Work out the finished part from the listing and answer in its coordinate system (mm). Face numbers are marked on the shaded views. A direction names the side the tool comes from. Coordinates: 2 decimals unless noted, no trailing zeros. Write each loop counter-clockwise with the first axis right and the second up, starting at its lowest first coordinate (ties: lowest second). Pieces come first, ordered by that corner, then holes. Notation, with made-up numbers: (-25, -35) - (12, -35) arc R17 cw to (12, -14) - close; hole circle Ø2 at (76.25, 65). An arc over 180 degrees is marked (long way). Use one line per item in the form item = value. Start each with the question number.
Item 1: A cutting plane is placed at B-B (y = 8). Write down the section's boundary in (x, z), then the cut area to 3 significant figures.
Item 2: Given pin 1 (5 mm diameter, centred on y = 4, z = 0.5, fed in from +X); pin 2 (5 mm diameter, centred on x = -0.5, y = 9, fed in from -Z); pin 3 (2 mm diameter, centred on y = 12.5, z = -3, fed in from +X), each flat-ended and moving along its own axis, determine where each tip first touches the part or whether it passes through.
Item 3: Consider probe 1 along Y at (x, z) = (-1.5, -3); probe 2 along Y at (x, z) = (0, 0.75); probe 3 along X at (y, z) = (6, -1.5). Determine where each line is inside the solid, lowest interval first.
Item 4: Determine the mould class of the marked faces 4, 5, 6 and 7 for opening direction X: released by +X, released by -X, zero draft, split by the parting line, or undercut.
Item 5: For the marked faces 1, 2 and 3, determine the directions among +Z, -Z, +X, -X, +Y, -Y from which every point of the face is accessible in a straight line to the end or side of a thin tool.
Item 6: A cutting plane is placed at A-A (z = 0). Write down the section's boundary in (x, y).
from build123d import *

# Parameters (mm, degrees)
SKETCH2_R           = 2.5
BOSS_EXTRUDE1_DEPTH = 30
SKETCH3_R           = 4.25
BOSS_EXTRUDE2_DEPTH = 5
FILLET1_R           = 0.4
CHAMFER1_SIZE       = 0.5
CUT_EXTRUDE1_DEPTH  = 2.5


with BuildPart() as part:
    # Sketch2 → Boss-Extrude1 (new body)
    with BuildSketch(Plane(origin=(0, 0, 0), x_dir=(1, 0, 0), z_dir=(0, 1, 0))):
        with Locations(Location((0, 0, 0), (0, 0, 270))):
            Circle(SKETCH2_R)
    extrude(amount=BOSS_EXTRUDE1_DEPTH)

    # Sketch3 → Boss-Extrude2 (add)
    with BuildSketch(Plane(origin=(0, 0, 0), x_dir=(1, 0, 0), z_dir=(0, 1, 0))):
        with Locations(Location((0, 0, 0), (0, 0, 270))):
            Circle(SKETCH3_R)
    extrude(amount=-BOSS_EXTRUDE2_DEPTH)

    # Fillet1
    fillet1_edges = [part.edges().sort_by_distance(p)[0] for p in [
        (0, 0, -2.5),
    ]]
    fillet(fillet1_edges, radius=FILLET1_R)

    # Chamfer1
    chamfer1_edges = [part.edges().sort_by_distance(p)[0] for p in [
        (0, 30, -2.5),
        (0, -5, -4.25),
    ]]
    chamfer(chamfer1_edges, length=CHAMFER1_SIZE)

    # Sketch4 → Cut-Extrude1 (cut)
    with BuildSketch(Plane.XZ.offset(5)):
        Polygon((0, 2.309401077), (-2, 1.154700538), (-2, -1.154700538), (0, -2.309401077), (2, -1.154700538), (2, 1.154700538), align=None)
    extrude(amount=-CUT_EXTRUDE1_DEPTH, mode=Mode.SUBTRACT)


solid = part.part
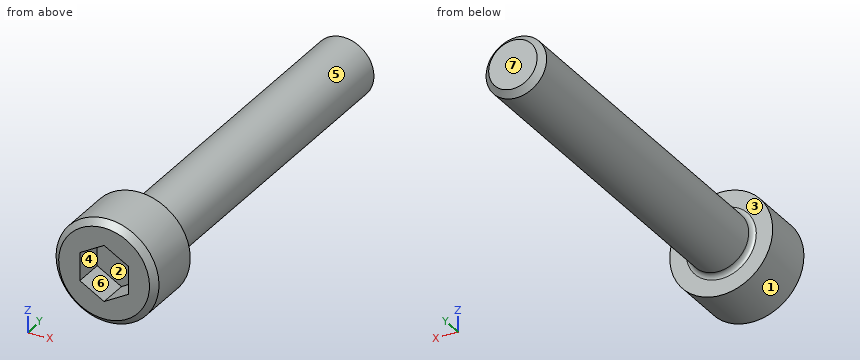
Answer:
q1.outline = circle Ø5 at (0, 0)
q1.area = 19.6 mm²
q2.pin_1 = 2.5
q2.pin_2 = -2.5
q2.pin_3 = 1.5
q3.probe_1 = -5 to 0
q3.probe_2 = -2.5 to 30
q3.probe_3 = -2 to 2
q4.face_4 = undercut
q4.face_5 = split by the parting line
q4.face_6 = undercut
q4.face_7 = zero draft
q5.face_1 = +Y, -Y
q5.face_2 = -Y
q5.face_3 = +Y
q6.outline = (-4.25, -4.5) - (-3.75, -5) - (-2, -5) - (-2, -2.5) - (2, -2.5) - (2, -5) - (3.75, -5) - (4.25, -4.5) - (4.25, 0) - (2.9, 0) arc R0.4 cw to (2.5, 0.4) - (2.5, 29.5) - (2, 30) - (-2, 30) - (-2.5, 29.5) - (-2.5, 0.4) arc R0.4 cw to (-2.9, 0) - (-4.25, 0) - close
